from build123d import *

# Parameters (mm, degrees)
SKETCH2_W           = 88.519
SKETCH2_H           = 153.924
BOSS_EXTRUDE2_DEPTH = 12.7
SKETCH2_6_W         = 82.169
SKETCH2_6_H         = 147.574
CUT_EXTRUDE1_DEPTH  = 10.16
SKETCH3_R           = 2.38125
CUT_EXTRUDE2_DEPTH  = 129.54
SKETCH4_W           = 88.519
SKETCH4_H           = 12.447800228
BOSS_EXTRUDE3_DEPTH = 6.35
FILLET1_R           = 2.54


with BuildPart() as part:
    # Sketch2 → Boss-Extrude2 (new body)
    with BuildSketch(Plane.XY):
        with Locations((41.0845, 73.787)):
            Rectangle(SKETCH2_W, SKETCH2_H)
    extrude(amount=BOSS_EXTRUDE2_DEPTH)

    # Sketch2<6> → Cut-Extrude1 (cut)
    with BuildSketch(Plane.XY):
        with Locations((41.0845, 73.787)):
            Rectangle(SKETCH2_6_W, SKETCH2_6_H)
    extrude(amount=CUT_EXTRUDE1_DEPTH, mode=Mode.SUBTRACT)

    # Sketch3 → Cut-Extrude2 (cut)
    with BuildSketch(Plane(origin=(85.344, 0, 0), x_dir=(0, 0, -1), z_dir=(1, 0, 0))):
        with Locations((-6.35, 6.217998886)):
            Circle(SKETCH3_R)
    extrude(amount=-CUT_EXTRUDE2_DEPTH, mode=Mode.SUBTRACT)

    # Sketch4 → Boss-Extrude3 (add)
    with BuildSketch(Plane.XZ.offset(3.175)):
        with Locations((41.0845, 6.223900114)):
            Rectangle(SKETCH4_W, SKETCH4_H)
    extrude(amount=BOSS_EXTRUDE3_DEPTH)

    # Fillet1
    fillet1_edges = [part.edges().sort_by_distance(p)[0] for p in [
        (-3.175, -9.525, 6.223900114),
        (85.344, -9.525, 6.223900114),
        (-3.175, 150.749, 6.35),
        (85.344, 150.749, 6.35),
    ]]
    fillet(fillet1_edges, radius=FILLET1_R)


solid = part.part
For this review, take the finished solid that the model builds, in its own axes (mm). A direction names the side the tool comes from. Coordinates: 2 decimals unless noted, no trailing zeros. Order: outer loops, then holes, each group sorted by start corner. A loop starts at its lowest first (then second) coordinate and runs counter-clockwise, first axis right, second up. Notation, with made-up numbers: (22, 41) -> (39, 41) arc R24 cw to (39, 54) -> close; hole circle Ø2 at (53.25, -29.5). An arc over 180 degrees is marked (long way). Return JSON: item names as keys, results as strings.
1. Machinability: for faces 1 (the flat face through (41, 147.574, 5)), 2 (the flat face through (-3.175, 72, 6)), 3 (the flat face through (40, -6, 12.448)), which of the approach directions +Z, -Z, +X, -X, +Y, -Y give a long, thin tool a straight path to every point of the face, cutting with its end or side? Answer none if there is none.
Answer block:
{"face 1": "-Z", "face 2": "+Z, -Z, -X, +Y, -Y", "face 3": "+Z, +X, -X, -Y"}
2. We need section A-A on z = 6.35. Write out the cut boundary in (x, y) (3 decimals).
Answer block:
{"outline": "(-3.175, -6.985) arc R2.54 ccw to (-0.635, -9.525) -> (82.804, -9.525) arc R2.54 ccw to (85.344, -6.985) -> (85.344, 3.837) -> (82.169, 3.837) -> (82.169, 0) -> (0, 0) -> (0, 3.837) -> (-3.175, 3.837) -> close; (-3.175, 8.599) -> (0, 8.599) -> (0, 147.574) -> (82.169, 147.574) -> (82.169, 8.599) -> (85.344, 8.599) -> (85.344, 148.209) arc R2.54 ccw to (82.804, 150.749) -> (-0.635, 150.749) arc R2.54 ccw to (-3.175, 148.209) -> close"}
3. We need section C-C on x = 19.5. Write out the cut boundary in (y, z) (3 decimals).
Answer block:
{"outline": "(-9.525, 0) -> (0, 0) -> (0, 10.16) -> (147.574, 10.16) -> (147.574, 0) -> (150.749, 0) -> (150.749, 12.7) -> (-3.175, 12.7) -> (-3.175, 12.448) -> (-9.525, 12.448) -> close"}
4. For line 1 (X direction, y = 45, z = 2.75) (3 decimals); line 2 (Y direction, x = 63.5, z = 6.25) (3 decimals); line 3 (Y direction, x = -0.8, z = 6.35), list the stretches that pass through material, from the lowest coordinate up. Write a range as from..to.
Answer block:
{"line 1": "-3.175..0, 82.169..85.344", "line 2": "-9.525..0, 147.574..150.749", "line 3": "-9.52..3.84, 8.6..150.74"}
5. The part is to be moulded in two halves that separate along Y. For faces 4 (the flat face through (85.344, 72, 6)), 5 (the flat face through (41, 0, 5)), 6 (the flat face through (41, -9.525, 6)), say which applies: +Y half, -Y half, draft (parallel to the pull), parting line (faces both ways), or undercut.
Answer block:
{"face 4": "draft", "face 5": "undercut", "face 6": "-Y half"}
6. We need section B-B on y = 108.5. Write out the cut boundary in (x, z) (3 decimals).
Answer block:
{"outline": "(-3.175, 0) -> (0, 0) -> (0, 10.16) -> (82.169, 10.16) -> (82.169, 0) -> (85.344, 0) -> (85.344, 12.7) -> (-3.175, 12.7) -> close"}
7. For pin 1 Ø12 at (x, y) = (48.5, 30.5) entering from -Z; pin 2 Ø5 at (x, y) = (21, -7) entering from +Z, all flat-tipped, find the tip position at first contact; note any pin that passes through.
Answer block:
{"pin 1": "z = 10.16", "pin 2": "z = 12.45"}
